Design review of the part built by this model. Coordinates are the model's own, in mm. Give positions to 0.01 mm unless a question says otherwise; leave off trailing zeros. Write each loop counter-clockwise with the first axis right and the second up, starting at its lowest first coordinate (ties: lowest second). Pieces come first, ordered by that corner, then holes. Notation, with made-up numbers: M -37,20.5 L 8,20.5 A20 ccw 8,30.5 Z; hole C -4,56 d9. An arc over 180 degrees is marked long. Use a Markdown table: item, result. Add a question column.
```python
from build123d import *

# Parameters (mm, degrees)
SKETCH1_W             = 69.85
SKETCH1_H             = 12.7
BOSS_EXTRUDE1_DEPTH   = 6.35
M6X1_0_TAPPED_HOLE1_D = 5
FILLET1_R             = 3.175


with BuildPart() as part:
    # Sketch1 → Boss-Extrude1 (new body)
    with BuildSketch(Plane(origin=(0, 0, 0), x_dir=(1, 0, 0), z_dir=(0, 1, 0))):
        with Locations((34.925, 0)):
            Rectangle(SKETCH1_W, SKETCH1_H)
    extrude(amount=BOSS_EXTRUDE1_DEPTH)

    # M6x1.0 Tapped Hole1 (through all)
    with Locations(Plane(origin=(0, 6.35, 0), x_dir=(1, 0, 0), z_dir=(0, 1, 0))):
        with Locations((4.7625, 0), (23.8125, 0), (65.0875, 0)):
            Hole(M6X1_0_TAPPED_HOLE1_D / 2)

    # Fillet1
    fillet1_edges = [part.edges().sort_by_distance(p)[0] for p in [
        (69.85, 3.175, -6.35),
        (69.85, 3.175, 6.35),
    ]]
    fillet(fillet1_edges, radius=FILLET1_R)


solid = part.part
```
(1) Add section B-B on y = 3.5. Give the number of separate pieces and of enclosed holes in the cut face, then the cut area to 3 significant figures.
(2) The part is to be moulded in two halves that separate along Z. For faces 1 (the flat face through (69.85, 3, 0)), 2 (the cylindrical face through (2.378, 3.131, -0.751)), 3 (the flat face through (33, 3, -6.35)), say which applies: released by +Z, released by -Z, zero draft, split by the parting line, or undercut.
(3) For pin 1 (3 mm diameter, centred on x = 44.5, z = 3.5, fed in from -Y), flat-tipped, find the tip position at first contact; note if it passes through.
(4) Wall thickness on L1, parallel to X at y = 4.25, z = 2; L2, parallel to X at y = 0.75, z = -1.5; L3, parallel to Z at x = 67, y = 4: over which ranges is each line inside the solid? List them lowest first.
(5) Add section C-C on x = 22. Give the boundary of the cut face in (y, z).
(6) Add section A-A on z = 0. Give the boundary of the cut face in (x, y), then the cut area to 3 significant figures.
From the geometry:
| question | item | result |
|---|---|---|
| 1 | separate pieces | 1 |
| 1 | enclosed holes | 3 |
| 1 | area | 824 mm^2 |
| 2 | face 1 | zero draft |
| 2 | face 2 | undercut |
| 2 | face 3 | released by -Z |
| 3 | pin 1 | stops at y = 0 |
| 4 | L1 | x = 0 to 3.26, 6.26 to 22.31, 25.31 to 63.59, 66.59 to 69.85 |
| 4 | L2 | x = 0 to 2.76, 6.76 to 21.81, 25.81 to 63.09, 67.09 to 69.85 |
| 4 | L3 | z = -6.33 to -1.61, 1.61 to 6.33 |
| 5 | outline | M 0,-6.35 L 6.35,-6.35 L 6.35,-1.72 L 0,-1.72 Z; M 0,1.72 L 6.35,1.72 L 6.35,6.35 L 0,6.35 Z |
| 6 | outline | M 0,0 L 2.26,0 L 2.26,6.35 L 0,6.35 Z; M 7.26,0 L 21.31,0 L 21.31,6.35 L 7.26,6.35 Z; M 26.31,0 L 62.59,0 L 62.59,6.35 L 26.31,6.35 Z; M 67.59,0 L 69.85,0 L 69.85,6.35 L 67.59,6.35 Z |
| 6 | area | 348 mm^2 |
